from build123d import *

# Parameters (mm, degrees)
SKETCH1_W           = 23
SKETCH1_H           = 20
BOSS_EXTRUDE1_DEPTH = 3
SKETCH2_W           = 3
SKETCH2_H           = 20
BOSS_EXTRUDE2_DEPTH = 20
CUT_EXTRUDE1_REACH  = 27.145
SKETCH3_R           = 2.5
CUT_EXTRUDE2_REACH  = 34.078
SKETCH4_R           = 2.5


with BuildPart() as part:
    # Sketch1 → Boss-Extrude1 (new body)
    with BuildSketch(Plane(origin=(0, 0, 0), x_dir=(0, 0, -1), z_dir=(1, 0, 0))):
        Rectangle(SKETCH1_W, SKETCH1_H)
    extrude(amount=BOSS_EXTRUDE1_DEPTH)

    # Sketch2 → Boss-Extrude2 (add)
    with BuildSketch(Plane(origin=(3, 0, 0), x_dir=(0, 0, -1), z_dir=(1, 0, 0))):
        with Locations((-10, 0)):
            Rectangle(SKETCH2_W, SKETCH2_H)
    extrude(amount=BOSS_EXTRUDE2_DEPTH)

    # Sketch3 → Cut-Extrude1 (cut, up to next)
    with BuildSketch(Plane(origin=(3, 0, 0), x_dir=(0, 0, -1), z_dir=(1, 0, 0)), mode=Mode.PRIVATE) as cut_extrude1_sk1:
        with Locations((1.5, 0)):
            Circle(SKETCH3_R)
    cut_extrude1_tool1 = extrude(cut_extrude1_sk1.sketch, amount=-CUT_EXTRUDE1_REACH, mode=Mode.PRIVATE) & part.part
    add(cut_extrude1_tool1.solids().sort_by_distance((3, 0, -1.5))[0], mode=Mode.SUBTRACT)

    # Sketch4 → Cut-Extrude2 (cut, up to next)
    with BuildSketch(Plane(origin=(0, 0, 8.5), x_dir=(-1, 0, 0), z_dir=(0, 0, -1)), mode=Mode.PRIVATE) as cut_extrude2_sk1:
        with Locations(Location((-13, 0, 0), (0, 0, 90))):
            Circle(SKETCH4_R)
    cut_extrude2_tool1 = extrude(cut_extrude2_sk1.sketch, amount=-CUT_EXTRUDE2_REACH, mode=Mode.PRIVATE) & part.part
    add(cut_extrude2_tool1.solids().sort_by_distance((13, 0, 8.5))[0], mode=Mode.SUBTRACT)


solid = part.part
Could you check a few things on this model? Use its own coordinates, in mm. A direction names the side the tool comes from. Give positions to 0.01 mm unless a question says otherwise; leave off trailing zeros. Write each loop counter-clockwise with the first axis right and the second up, starting at its lowest first coordinate (ties: lowest second). Pieces come first, ordered by that corner, then holes. Notation, with made-up numbers: (5, -3.5) -> (48, -3.5) arc R13 ccw to (48, 5.5) -> close; hole circle Ø3 at (-32, 6.5). An arc over 180 degrees is marked (long way). Answer as a JSON object with one key per item and string values.
Q1. Suppose I cut it at B-B on x = 13. Write out the boundary of the cut face in (y, z).
Taken from the geometry:
{"outline": "(-10, 8.5) -> (-2.5, 8.5) -> (-2.5, 11.5) -> (-10, 11.5) -> close; (2.5, 8.5) -> (10, 8.5) -> (10, 11.5) -> (2.5, 11.5) -> close"}
Q2. Suppose I cut it at C-C on y = 0. Write out the boundary of the cut face in (x, z).
Taken from the geometry:
{"outline": "(0, -11.5) -> (3, -11.5) -> (3, -4) -> (0, -4) -> close; (0, 1) -> (3, 1) -> (3, 8.5) -> (10.5, 8.5) -> (10.5, 11.5) -> (0, 11.5) -> close; (15.5, 8.5) -> (23, 8.5) -> (23, 11.5) -> (15.5, 11.5) -> close"}
Q3. Which directions (+Z, -Z, +X, -X, +Y, -Y) give clear straight access to the entire face, cutting with the end or side of a thin tool? Please do faces 1 (the flat face through (15, -2, 8.5)), 2 (the flat face through (23, 0, 10)).
Taken from the geometry:
{"face 1": "-Z, +X, +Y, -Y", "face 2": "+Z, -Z, +X, +Y, -Y"}
Q4. Will these pins go through, and if not, where does the flat tip stop? pin 1 Ø2 at (y, z) = (7, -6) entering from +X; pin 2 Ø8 at (x, y) = (11, -5.5) entering from -Z.
Taken from the geometry:
{"pin 1": "stops at x = 3", "pin 2": "stops at z = 8.5"}
Q5. Suppose I cut it at A-A on z = -1.5. Write out the boundary of the cut face in (x, y), then the cut area to 3 significant figures.
Taken from the geometry:
{"outline": "(0, -10) -> (3, -10) -> (3, -2.5) -> (0, -2.5) -> close; (0, 2.5) -> (3, 2.5) -> (3, 10) -> (0, 10) -> close", "area": "45.0 mm²"}
Q6. We'd pull the mould along X, two halves only. Please class faces 3 (the flat face through (3, 2, -4)), 4 (the cylindrical face through (10.56, -0.54, 9.98)), 5 (the flat face through (11, -2, 11.5)): released by +X, released by -X, zero draft, split by the parting line, or undercut.
Taken from the geometry:
{"face 3": "released by +X", "face 4": "undercut", "face 5": "zero draft"}
Q7. Suppose I cut it at D-D on z = 9. Write out the boundary of the cut face in (x, y).
Taken from the geometry:
{"outline": "(0, -10) -> (23, -10) -> (23, 10) -> (0, 10) -> close; hole circle Ø5 at (13, 0)"}
Q8. Please list where these lines run through material, in increasing order: L1, parallel to Y at x = 2, z = -1.5; L2, parallel to Z at x = 6.75, y = 2; L3, parallel to X at y = -5.5, z = 8.
Taken from the geometry:
{"L1": "y = -10 to -2.5, 2.5 to 10", "L2": "z = 8.5 to 11.5", "L3": "x = 0 to 3"}
